Check sheet for the modelled part. Datum: model origin and axes. Units: mm. Round coordinates to 2 decimals unless told otherwise and drop trailing zeros. Write each loop counter-clockwise with the first axis right and the second up, starting at its lowest first coordinate (ties: lowest second). Pieces come first, ordered by that corner, then holes. Notation, with made-up numbers: M -9.75,-1.75 L 4.25,-1.75 A15 cw 4.25,10.25 Z; hole C 86,53.25 d8. An arc over 180 degrees is marked long. Answer in a Markdown table with one row per item.
```python
from build123d import *

# Parameters (mm, degrees)
F1_DEPTH = 371.4496


with BuildPart() as f1:
    # F0 (on Top) → F1 (new body)
    with BuildSketch(Plane.XY):
        Polygon((0, 5.08), (0, 0), (7.62, 0), (7.62, 1.27), (1.27, 1.27), (1.27, 2.54), (2.54, 2.54), (2.54, 5.08), align=None)
    extrude(amount=F1_DEPTH)

    # F2: F1 across face


with BuildPart() as f1_1:
    add(f1.part)
    add(f1.part.mirror(Plane(origin=(7.62, 0.635, 185.7248), x_dir=(0, 1, 0), z_dir=(1, 0, 0))))


solid = f1_1.part
```
1. Scan lines: L1, parallel to Y at x = 2.25, z = 67; L2, parallel to X at y = 1.85, z = 330.5; L3, parallel to X at y = 2.75, z = 16.5. Record each from-to range of solid material in increasing order.
Found:
| item | result |
|---|---|
| L1 | y = 0 to 1.27, 2.54 to 5.08 |
| L2 | x = 0 to 1.27, 13.97 to 15.24 |
| L3 | x = 0 to 2.54, 12.7 to 15.24 |
2. Go/stop test with a flat-tipped pin: pin 1 (4 mm diameter, centred on x = 7, z = 146, fed in from +Y). Record where the tip stops, or that it passes through.
Found:
| item | result |
|---|---|
| pin 1 | stops at y = 1.27 |
3. Draft check along X on faces 1 (the face through (8, 1.27, 183)), 2 (the face through (8, 0, 183)). Enter one of: +X half, -X half, draft (parallel to the pull), parting line (faces both ways), or undercut.
Found:
| item | result |
|---|---|
| face 1 | undercut |
| face 2 | draft |
4. Section check A-A, the plane z = 194. Record the cut outline in (x, y).
Found:
| item | result |
|---|---|
| outline | M 0,0 L 15.24,0 L 15.24,5.08 L 12.7,5.08 L 12.7,2.54 L 13.97,2.54 L 13.97,1.27 L 1.27,1.27 L 1.27,2.54 L 2.54,2.54 L 2.54,5.08 L 0,5.08 Z |
5. Section check B-B, the plane x = 9.75. Record the cut outline in (y, z).
Found:
| item | result |
|---|---|
| outline | M 0,0 L 1.27,0 L 1.27,371.45 L 0,371.45 Z |
